Check sheet for the modelled part. Datum: model origin and axes. Units: mm. Round coordinates to 2 decimals unless told otherwise and drop trailing zeros. Order: outer loops, then holes, each group sorted by start corner. A loop starts at its lowest first (then second) coordinate and runs counter-clockwise, first axis right, second up.
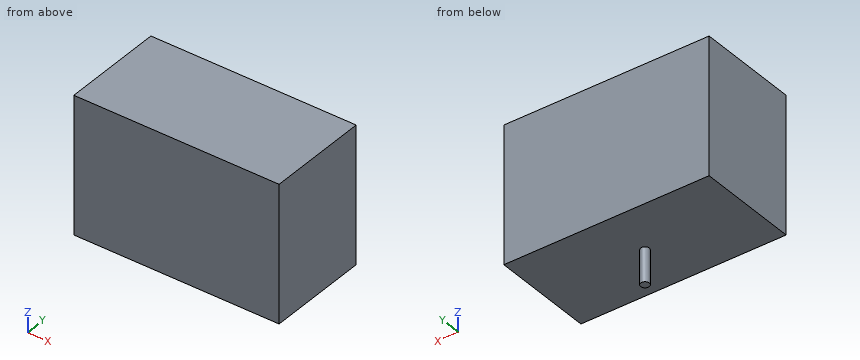
```python
from build123d import *

# Parameters (mm, degrees)
F0_W     = 152.4
F0_H     = 203.2
F1_DEPTH = 152.4
F2_R     = 6.35
F3_DEPTH = 50.8


with BuildPart() as f1:
    # F0 (on Front) → F1 (new body)
    with BuildSketch(Plane.XZ):
        with Locations((-76.2, 101.6)):
            Rectangle(F0_W, F0_H)
        with Locations((76.2, 101.6)):
            Rectangle(F0_W, F0_H)
    extrude(amount=F1_DEPTH)

    # F2 (on face) → F3 (join)
    with BuildSketch(Plane(origin=(0, 0, 0), x_dir=(1, 0, 0), z_dir=(0, 0, -1))):
        with Locations((0, 76.2)):
            Circle(F2_R)
    extrude(amount=F3_DEPTH)


solid = f1.part
```
Item 1: Scan lines: line 1 along Z through (x, y) = (-77.5, -68.5); line 2 along X through (y, z) = (-77, -16). Record each from-to range of solid material in increasing order.
Answer:
line 1: z = 0 to 203.2
line 2: x = -6.3 to 6.3
Item 2: Sectioned sample at D-D (x = 68.5). Record the cut outline in (y, z), and give its area (3 significant figures).
Answer:
outline: (-152.4, 0) - (0, 0) - (0, 203.2) - (-152.4, 203.2) - close
area: 31,000 mm2
Item 3: Sectioned sample at A-A (x = 0). Record the cut outline in (y, z), and give its area (3 significant figures).
Answer:
outline: (-152.4, 0) - (-82.55, 0) - (-82.55, -50.8) - (-69.85, -50.8) - (-69.85, 0) - (0, 0) - (0, 203.2) - (-152.4, 203.2) - close
area: 31,600 mm2
Item 4: Sectioned sample at B-B (y = -76.2). Record the cut outline in (x, z).
Answer:
outline: (-152.4, 0) - (-6.35, 0) - (-6.35, -50.8) - (6.35, -50.8) - (6.35, 0) - (152.4, 0) - (152.4, 203.2) - (-152.4, 203.2) - close
Item 5: Sectioned sample at C-C (z = -13). Record the cut outline in (x, y).
Answer:
outline: circle Ø12.7 at (0, -76.2)
Item 6: Go/stop test with flat-tipped pins: P1, Ø10, axis at x = -65, z = -6.5, coming from the +Y side; P2, Ø6, axis at x = 18.5, y = -90, coming from the -Z side. Record where each tip stops, or that it passes through.
Answer:
P1: passes through
P2: stops at z = 0
